Design review of the part built by this model. Coordinates are the model's own, in mm. A direction names the side the tool comes from. Give positions to 0.01 mm unless a question says otherwise; leave off trailing zeros. Loops run counter-clockwise (first coordinate to the right, second up) from the corner with the lowest first, then second, coordinate; pieces in that order, holes last. Notation, with made-up numbers: (-10.5, 14) - (41.5, 14) arc R24 ccw to (41.5, 43) - close; hole circle Ø4 at (82.5, 67.5). An arc over 180 degrees is marked (long way). Put each result on its own line as item: value. Start each with the question number.
```python
from build123d import *

# Parameters (mm, degrees)
F0_R      = 3.25
F1_DEPTH  = 15
F2_R      = 1.75
F3_DEPTH  = 8
F5_R      = 1.75
F6_DEPTH  = 2
F8_R      = 1.75
F9_DEPTH  = 2
F10_R     = 0.5
F11_DEPTH = 1


with BuildPart() as f1:
    # F0 (on Top) → F1 (new body)
    with BuildSketch(Plane.XY):
        Circle(F0_R)
    extrude(amount=F1_DEPTH)

    # F2 (on face) → F3 (cut)
    with BuildSketch(Plane(origin=(0, 0, 0), x_dir=(1, 0, 0), z_dir=(0, 0, -1))):
        Circle(F2_R)
    extrude(amount=-F3_DEPTH, mode=Mode.SUBTRACT)

    # F5 (on offset) → F6 (cut)
    with BuildSketch(Plane(origin=(0, 0, 9), x_dir=(1, 0, 0), z_dir=(0, 0, -1))):
        Circle(F5_R)
    extrude(amount=-F6_DEPTH, mode=Mode.SUBTRACT)

    # F8 (on offset) → F9 (cut)
    with BuildSketch(Plane(origin=(0, 0, 12), x_dir=(1, 0, 0), z_dir=(0, 0, -1))):
        Circle(F8_R)
    extrude(amount=-F9_DEPTH, mode=Mode.SUBTRACT)

    # F10 (on offset) → F11 (cut)
    with BuildSketch(Plane(origin=(0, 0, 12), x_dir=(1, 0, 0), z_dir=(0, 0, -1))):
        with Locations((-1, -0.5)):
            Circle(F10_R)
        with Locations((1, -0.5)):
            Circle(F10_R)
        with Locations((0, 1)):
            Circle(F10_R)
    extrude(amount=F11_DEPTH, mode=Mode.SUBTRACT)


solid = f1.part
```
Item 1: Mouldability with a two-part tool opening along Y and no side actions: class faces 4 (the flat face through (0, 0, 9)), 5 (the flat face through (1.4, -1.4, 0)), 6 (the cylindrical face through (-2.579, -1.978, 7.395)) as pulls with the +Y half, pulls with the -Y half, needs draft (parallel to the pull), parting line crosses it, or undercut.
Item 2: Consider section A-A (y = 0.5). State the section outline as (x, z) points, plus the area to 3 significant figures.
Item 3: Consider section D-D (z = 6.25). State the section outline as (x, y) points, plus the area to 3 significant figures.
Item 4: Consider section C-C (y = -0.75). State the section outline as (x, z) points.
Item 5: Machinability: for faces 1 (the cylindrical face through (-0.108, -0.512, 11.507)), 2 (the flat face through (0, 0, 15)), 3 (the cylindrical face through (1.617, 0.67, 3.944)), which of the approach directions +Z, -Z, +X, -X, +Y, -Y give a long, thin tool a straight path to every point of the face, cutting with its end or side? Answer none if there is none.
Item 6: For P1, Ø1, axis at x = 0.5, y = 1, coming from the -Z side, flat-tipped, find the tip position at first contact; note if it passes through.
Item 7: For L1, parallel to Y at x = 0, z = 3; L2, parallel to X at y = 0.5, z = 11.3; L3, parallel to Y at x = 0, z = 11.3, list the stretches that pass through material, from the lowest coordinate up. Write a range as from..to.
Item 8: Consider section B-B (x = 0). State the section outline as (y, z) points, plus the area to 3 significant figures.
Geometry says:
1. face 4: undercut
1. face 5: needs draft
1. face 6: parting line crosses it
2. outline: (-3.21, 0) - (-1.68, 0) - (-1.68, 8) - (1.68, 8) - (1.68, 0) - (3.21, 0) - (3.21, 15) - (-3.21, 15) - close; (-0.5, 11) - (0.5, 11) - (0.5, 12) - (-0.5, 12) - close; hole (-1.68, 9) - (1.68, 9) - (1.68, 11) - (1.5, 11) - (1.5, 12) - (1.68, 12) - (1.68, 14) - (-1.68, 14) - (-1.68, 12) - (-1.5, 12) - (-1.5, 11) - (-1.68, 11) - close
2. area: 54.1 mm2
3. outline: circle Ø6.5 at (0, 0); hole circle Ø3.5 at (0, 0)
3. area: 23.6 mm2
4. outline: (-3.16, 0) - (-1.58, 0) - (-1.58, 8) - (1.58, 8) - (1.58, 0) - (3.16, 0) - (3.16, 15) - (-3.16, 15) - close; hole (-1.58, 9) - (1.58, 9) - (1.58, 11) - (0.43, 11) - (0.43, 12) - (1.58, 12) - (1.58, 14) - (-1.58, 14) - (-1.58, 12) - (-0.43, 12) - (-0.43, 11) - (-1.58, 11) - close
5. face 1: none
5. face 2: +Z, +X, -X, +Y, -Y
5. face 3: -Z
6. P1: stops at z = 8
7. L1: y = -3.25..-1.75, 1.75..3.25
7. L2: x = -3.21..-1.5, -0.5..0.5, 1.5..3.21
7. L3: y = -3.25..-1.5, -0.5..3.25
8. outline: (-3.25, 0) - (-1.75, 0) - (-1.75, 8) - (1.75, 8) - (1.75, 0) - (3.25, 0) - (3.25, 15) - (-3.25, 15) - close; hole (-1.75, 9) - (1.75, 9) - (1.75, 11) - (-0.5, 11) - (-0.5, 12) - (1.75, 12) - (1.75, 14) - (-1.75, 14) - (-1.75, 12) - (-1.5, 12) - (-1.5, 11) - (-1.75, 11) - close
8. area: 54.5 mm2
